Geometry: final body of the model. Coordinates: model frame, mm. A direction names the side the tool comes from. Give positions to 0.01 mm unless a question says otherwise; leave off trailing zeros. Order: outer loops, then holes, each group sorted by start corner. A loop starts at its lowest first (then second) coordinate and runs counter-clockwise, first axis right, second up. Notation, with made-up numbers: (27, 14.25) -> (59, 14.25) arc R17 ccw to (59, 34.25) -> close; hole circle Ø6 at (-17, -38). An arc over 180 degrees is marked (long way). Write item = value, one per line.
```python
from build123d import *

# Parameters (mm, degrees)
ESBO_O1_W                      = 33
ESBO_O1_H                      = 45
RESSALTO_EXTRUS_O1_DEPTH       = 20
FURO_DE_DI_METRO_15_0_15_1_D   = 15
FURO_ROSCADO_DE_M10X1_51_D     = 8.5
FURO_ROSCADO_DE_M10X1_51_DEPTH = 17.446342369
FURO_ROSCADO_DE_M10X1_51_TIP   = 2.553657631
ESBO_O6_W                      = 6.5
ESBO_O6_H                      = 13
CORTE_EXTRUS_O1_DEPTH          = 63.42795848


with BuildPart() as part:
    # Esboço1 → Ressalto-extrusão1 (new, symmetric)
    with BuildSketch(Plane(origin=(0, 0, 0), x_dir=(1, 0, 0), z_dir=(0, 1, 0))):
        with Locations((0, 22.5)):
            Rectangle(ESBO_O1_W, ESBO_O1_H)
    extrude(amount=RESSALTO_EXTRUS_O1_DEPTH, both=True)

    # Furo de diâmetro Ø15.0 (15)1 (through all)
    with Locations(Plane(origin=(0, 20, 0), x_dir=(1, 0, 0), z_dir=(0, 1, 0))):
        with Locations((0, 13.15)):
            Hole(FURO_DE_DI_METRO_15_0_15_1_D / 2)

    # Furo roscado de M10x1.51
    with Locations(Plane(origin=(0, 0, -45), x_dir=(-1, 0, 0), z_dir=(0, 0, -1))):
        with Locations((0, 0)):
            Hole(FURO_ROSCADO_DE_M10X1_51_D / 2, depth=FURO_ROSCADO_DE_M10X1_51_DEPTH)
            with Locations((0, 0, -(FURO_ROSCADO_DE_M10X1_51_DEPTH + FURO_ROSCADO_DE_M10X1_51_TIP / 2))):  # 118° drill point
                Cone(0, FURO_ROSCADO_DE_M10X1_51_D / 2, FURO_ROSCADO_DE_M10X1_51_TIP, mode=Mode.SUBTRACT)

    # Esboço6 → Corte-extrusão1 (cut, through all)
    with BuildSketch(Plane(origin=(0, 20, 0), x_dir=(1, 0, 0), z_dir=(0, 1, 0))):
        with Locations((-13.25, 34.5)):
            Rectangle(ESBO_O6_W, ESBO_O6_H)
        with Locations((13.25, 34.5)):
            Rectangle(ESBO_O6_W, ESBO_O6_H)
    extrude(amount=-CORTE_EXTRUS_O1_DEPTH, mode=Mode.SUBTRACT)


solid = part.part
```
1) Reachability of faces 1 (the face through (-13, 0, -41)), 2 (the face through (2.285, 3.584, -36.155)), 3 (the face through (13, 0, -28)), 4 (the face through (0, 5, -45)) from +Z, -Z, +X, -X, +Y, -Y: full face, straight path, thin tool, end or side. Return the list, or none.
Check sheet entries:
face_1 = -X, +Y, -Y
face_2 = -Z
face_3 = +X, +Y, -Y
face_4 = -Z, +X, -X, +Y, -Y
2) Section query D-D (z = -34). Output: boundary loops of the cut face in (x, y), plus the area to 3 significant figures.
Check sheet entries:
outline = (-10, -20) -> (10, -20) -> (10, 20) -> (-10, 20) -> close; hole circle Ø8.5 at (0, 0)
area = 743 mm²
3) Mould query, pull axis Z, two halves, no side actions, for faces 5 (the face through (5.528, -0.28, -18.219)), 6 (the face through (0, 0, 0)), 7 (the face through (-16.5, 0, -43)), 8 (the face through (0.16, -0.721, -25.443)). Classes: +Z half, -Z half, draft (parallel to the pull), parting line (faces both ways), or undercut.
Check sheet entries:
face_5 = undercut
face_6 = +Z half
face_7 = draft
face_8 = -Z half
4) Line query: line 1 (Y direction, x = 0, z = -35.75); line 2 (Z direction, x = 0, y = -9); line 3 (Z direction, x = 14, y = 13). Output: solid intervals per line, ascending. Write a range as from..to.
Check sheet entries:
line_1 = -20..-4.25, 4.25..20
line_2 = -45..-20.65, -5.65..0
line_3 = -45..-41, -28..0
5) Section query C-C (x = 14). Output: boundary loops of the cut face in (y, z).
Check sheet entries:
outline = (-20, -45) -> (20, -45) -> (20, -41) -> (-20, -41) -> close; (-20, -28) -> (20, -28) -> (20, 0) -> (-20, 0) -> close
6) First-contact query: P1, Ø9, axis at x = 0, z = -13.15, coming from the +Y side; P2, Ø3, axis at y = 14.5, z = -36, coming from the +X side; P3, Ø3, axis at y = 2, z = -30.5, coming from the -X side; P4, Ø5, axis at x = 0, y = 0, coming from the +Z side. Flat tips, straight axial feed; report the tip coordinate or a pass-through.
Check sheet entries:
P1 = through
P2 = 10
P3 = -10
P4 = 0
7) Section query B-B (y = -14.5). Output: boundary loops of the cut face in (x, z), plus the area to 3 significant figures.
Check sheet entries:
outline = (-16.5, -45) -> (16.5, -45) -> (16.5, -41) -> (10, -41) -> (10, -28) -> (16.5, -28) -> (16.5, 0) -> (-16.5, 0) -> (-16.5, -28) -> (-10, -28) -> (-10, -41) -> (-16.5, -41) -> close; hole circle Ø15 at (0, -13.15)
area = 1,140 mm²
8) Section query A-A (z = -13.15). Output: boundary loops of the cut face in (x, y), plus the area to 3 significant figures.
Check sheet entries:
outline = (-16.5, -20) -> (-7.5, -20) -> (-7.5, 20) -> (-16.5, 20) -> close; (7.5, -20) -> (16.5, -20) -> (16.5, 20) -> (7.5, 20) -> close
area = 720 mm²
